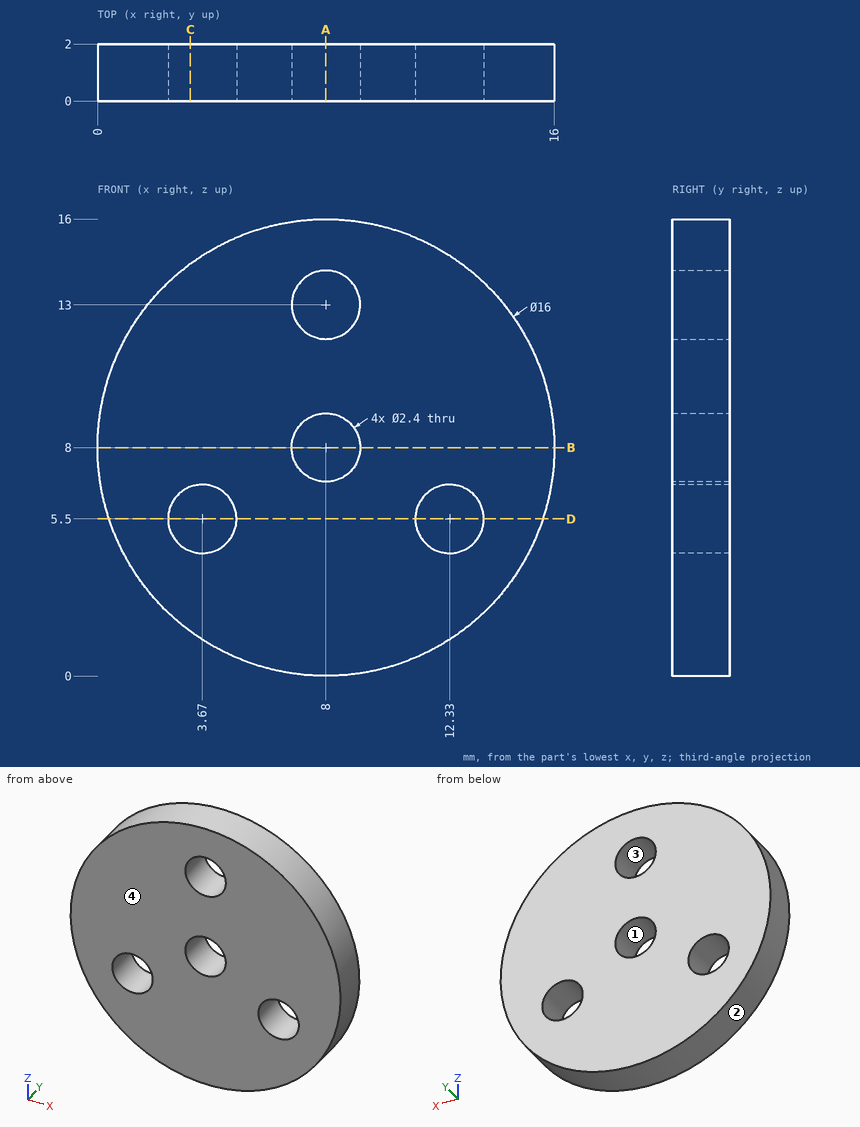
The figure shows three views and two pictorial views of one solid part (mm, origin at its lowest corner). Answer the questions. Coordinates: 2 decimals unless noted, no trailing zeros. Loops run counter-clockwise (first coordinate to the right, second up) from the corner with the lowest first, then second, coordinate; pieces in that order, holes last. Notation, with made-up numbers: (34, 27.5) - (84, 27.5) arc R27 ccw to (84, 46.5) - close; hole circle Ø7 at (84, -19). An arc over 180 degrees is marked (long way). Use a Markdown table: item, result. Add a question column.
1) The part is cut by section D-D, the plane z = 5.5. Give the vertices of the cut face in (x, y), and give its area (3 significant figures).
2) Given pin 1 (1 mm diameter, centred on x = 4, y = 0.5, fed in from +Z), flat-ended and moving along its own axis, determine where the tip first touches the part or whether it passes through.
3) The mould has two halves that part along Z. Classify the marked faces 1, 2, 3 and 4: released by +Z, released by -Z, zero draft, split by the parting line, or undercut.
4) The part is cut by section B-B, the plane z = 8. Give the vertices of the cut face in (x, y).
5) Find the intervals of material crossed by line 1 (Z direction, x = 7, y = 0.5); line 2 (X direction, y = 1.2, z = 5.5); line 3 (X direction, y = 1, z = 6), in increasing order.
6) The part is cut by section C-C, the plane x = 3.25. Give the vertices of the cut face in (y, z).
7) The part is cut by section A-A, the plane x = 8. Give the vertices of the cut face in (y, z).
Here are the results:
| question | item | result |
|---|---|---|
| 1 | outline | (0.4, 0) - (2.47, 0) - (2.47, 2) - (0.4, 2) - close; (4.87, 0) - (11.13, 0) - (11.13, 2) - (4.87, 2) - close; (13.53, 0) - (15.6, 0) - (15.6, 2) - (13.53, 2) - close |
| 1 | area | 20.8 mm^2 |
| 2 | pin 1 | stops at z = 15.19 |
| 3 | face 1 | undercut |
| 3 | face 2 | split by the parting line |
| 3 | face 3 | undercut |
| 3 | face 4 | zero draft |
| 4 | outline | (0, 0) - (6.8, 0) - (6.8, 2) - (0, 2) - close; (9.2, 0) - (16, 0) - (16, 2) - (9.2, 2) - close |
| 5 | line 1 | z = 0.06 to 7.34, 8.66 to 12.34, 13.66 to 15.94 |
| 5 | line 2 | x = 0.4 to 2.47, 4.87 to 11.13, 13.53 to 15.6 |
| 5 | line 3 | x = 0.25 to 2.58, 4.76 to 11.24, 13.42 to 15.75 |
| 6 | outline | (0, 1.56) - (2, 1.56) - (2, 4.38) - (0, 4.38) - close; (0, 6.62) - (2, 6.62) - (2, 14.44) - (0, 14.44) - close |
| 7 | outline | (0, 0) - (2, 0) - (2, 6.8) - (0, 6.8) - close; (0, 9.2) - (2, 9.2) - (2, 11.8) - (0, 11.8) - close; (0, 14.2) - (2, 14.2) - (2, 16) - (0, 16) - close |
